The figure shows three views and two pictorial views of one solid part (mm, origin at its lowest corner). Answer the questions. A direction names the side the tool comes from. Give positions to 0.01 mm unless a question says otherwise; leave off trailing zeros. Write each loop counter-clockwise with the first axis right and the second up, starting at its lowest first coordinate (ties: lowest second). Pieces come first, ordered by that corner, then holes. Notation, with made-up numbers: (46, -36.5) - (87, -36.5) arc R27 cw to (87, -16.5) - close; hole circle Ø9 at (33.25, 7). An arc over 180 degrees is marked (long way). Use a Markdown table: item, result. Add a question column.
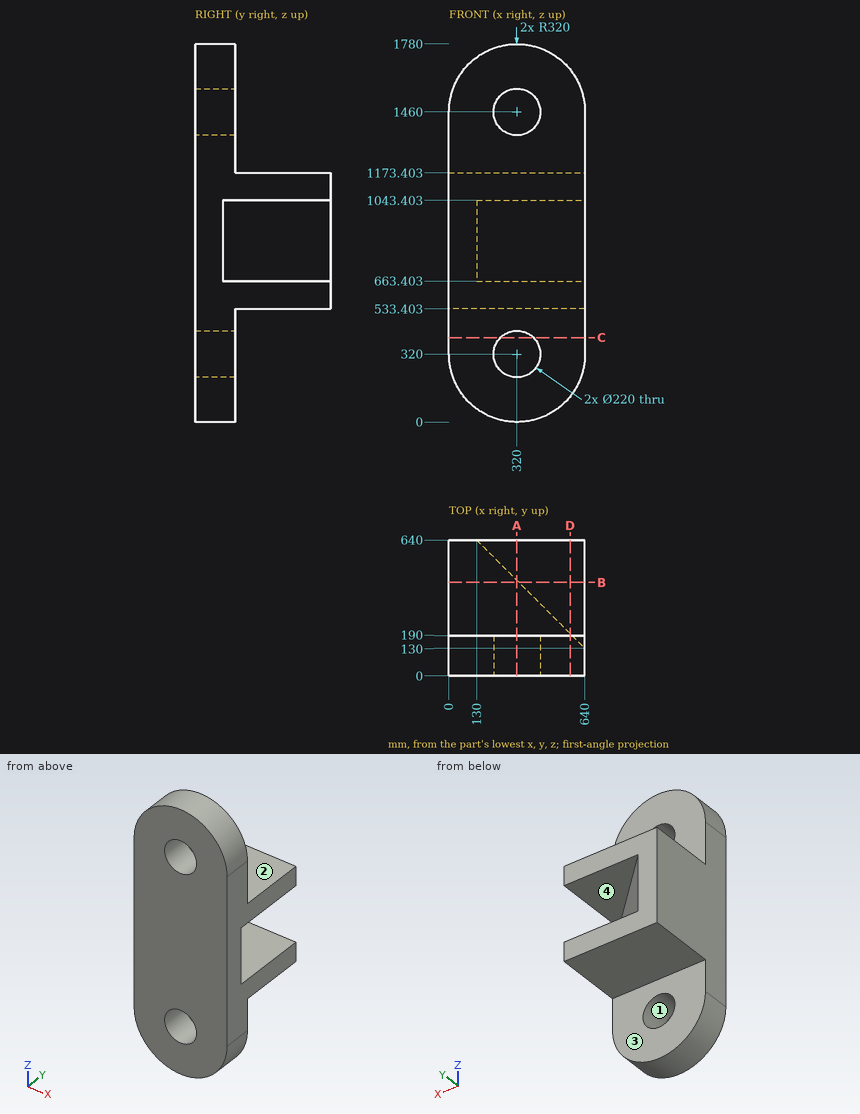
1. Which of the six approach directions +Z, -Z, +X, -X, +Y, -Y give full straight-line access (tool end or side, diameter ignored) to the marked faces 1, 2, 3 and 4?
2. The part is cut by section B-B (y = 441). Give the vertices of the cut face in (x, z).
3. The part is cut by section C-C (z = 397). Give the vertices of the cut face in (x, y) (1 decimal), and give its area (4 significant figures).
4. The part is cut by section D-D (x = 570). Give the vertices of the cut face in (y, z).
5. The part is cut by section A-A (x = 320). Give the vertices of the cut face in (y, z).
6. Given P1, Ø2, axis at x = 124.5, y = 124.5, coming from the +Z side (1 decimal); P2, Ø6, axis at x = 144, z = 358, coming from the +Y side; P3, Ø4, axis at x = 71.5, z = 473.5, coming from the -Y side; P4, Ø3, axis at x = 112, y = 187.5, coming from the +Z side (1 decimal), each flat-ended and moving along its own axis, determine where each tip first touches the part or whether it passes through.
7. Consider L1, parallel to Z at x = 315, y = 99.5; L2, parallel to X at y = 60.5, z = 1460; L3, parallel to Z at x = 397, y = 35 (1 decimal). Determine where each line is inside the solid, lowest interval first. Write a range as [from, to].
Check values:
| question | item | result |
|---|---|---|
| 1 | face 1 | +Y, -Y |
| 1 | face 2 | +Z, +X, -X, +Y |
| 1 | face 3 | -Z, +X, -X, +Y |
| 1 | face 4 | +X, +Y |
| 2 | outline | (0, 533.4) - (640, 533.4) - (640, 663.4) - (329, 663.4) - (329, 1043.4) - (640, 1043.4) - (640, 1173.4) - (0, 1173.4) - close |
| 3 | outline | (0, 0) - (241.4, 0) - (241.4, 190) - (0, 190) - close; (398.6, 0) - (640, 0) - (640, 190) - (398.6, 190) - close |
| 3 | area | 91,750 mm2 |
| 4 | outline | (0, 120.25) - (190, 120.25) - (190, 533.4) - (640, 533.4) - (640, 663.4) - (200, 663.4) - (200, 1043.4) - (640, 1043.4) - (640, 1173.4) - (190, 1173.4) - (190, 1659.75) - (0, 1659.75) - close |
| 5 | outline | (0, 0) - (190, 0) - (190, 210) - (0, 210) - close; (0, 430) - (190, 430) - (190, 533.4) - (640, 533.4) - (640, 663.4) - (450, 663.4) - (450, 1043.4) - (640, 1043.4) - (640, 1173.4) - (190, 1173.4) - (190, 1350) - (0, 1350) - close; (0, 1570) - (190, 1570) - (190, 1780) - (0, 1780) - close |
| 6 | P1 | stops at z = 1714.1 |
| 6 | P2 | stops at y = 190 |
| 6 | P3 | stops at y = 0 |
| 6 | P4 | stops at z = 1704.5 |
| 7 | L1 | z = [0.04, 210.11], [429.89, 1350.11], [1569.89, 1779.96] |
| 7 | L2 | x = [0, 210], [430, 640] |
| 7 | L3 | z = [9.4, 241.4], [398.6, 1381.4], [1538.6, 1770.6] |
